from build123d import *

# Parameters (mm, degrees)
CYLINDER001_R     = 1.5
CYLINDER001_DEPTH = 10
CYLINDER_R        = 1.5
CYLINDER_DEPTH    = 10
EXTRUDE_DEPTH     = 12
BOX_W             = 31
BOX_H             = 12.3
BOX_DEPTH         = 0.75


with BuildPart() as screw_hole2:
    # Cylinder001 → Cylinder001 (new body)
    with BuildSketch(Plane(origin=(12.27, 0, 0), x_dir=(1, 0, 0), z_dir=(0, 0, 1))):
        Circle(CYLINDER001_R)
    extrude(amount=CYLINDER001_DEPTH)


with BuildPart() as screw_hole1:
    # Cylinder → Cylinder (new body)
    with BuildSketch(Plane(origin=(-12.27, 0, 0), x_dir=(1, 0, 0), z_dir=(0, 0, 1))):
        Circle(CYLINDER_R)
    extrude(amount=CYLINDER_DEPTH)


with BuildPart() as extrude_body:
    # Sketch → Extrude (new body)
    with BuildSketch(Plane.XY):
        with BuildLine():
            Line((-6.770935, 4.5), (6.770935, 4.5))
            ThreePointArc((9.25, 1.677142), (8.649385, 3.649675), (6.770935, 4.5))
            Line((9.25, 1.677142), (8.729065, -2.322858))
            ThreePointArc((6.25, -4.5), (7.899675, -3.878449), (8.729065, -2.322858))
            Line((6.25, -4.5), (-6.25, -4.5))
            ThreePointArc((-8.729065, -2.322858), (-7.899675, -3.878449), (-6.25, -4.5))
            Line((-8.729065, -2.322858), (-9.25, 1.677142))
            ThreePointArc((-6.770935, 4.5), (-8.649385, 3.649675), (-9.25, 1.677142))
        make_face()
    extrude(amount=EXTRUDE_DEPTH)


with BuildPart() as db9_connector:
    # Box → Box (new body)
    with BuildSketch(Plane(origin=(-15.5, -6.13, 6), x_dir=(1, 0, 0), z_dir=(0, 0, 1))):
        with Locations((15.5, 6.15)):
            Rectangle(BOX_W, BOX_H)
    extrude(amount=BOX_DEPTH)

    # Fusion: union Extrude body
    add(extrude_body.part)

    # Cut: cut screw_hole1
    add(screw_hole1.part, mode=Mode.SUBTRACT)

    # Cut001: cut screw_hole2
    add(screw_hole2.part, mode=Mode.SUBTRACT)


solid = db9_connector.part
Here's how the part is built. I have some questions about the finished solid (model axes, mm). A direction names the side the tool comes from. Round coordinates to 2 decimals unless told otherwise and drop trailing zeros. Loops run counter-clockwise (first coordinate to the right, second up) from the corner with the lowest first, then second, coordinate; pieces in that order, holes last. Notation, with made-up numbers: (-1, -33.5) -> (23, -33.5) arc R26 cw to (23, -14.5) -> close; hole circle Ø2 at (-37, 48). An arc over 180 degrees is marked (long way). Write each question's results on one line, items separated by ' | '.
(1) If I drill on L1, parallel to X at y = 0, z = 6.35; L2, parallel to Y at x = -12.27, z = 6.4; L3, parallel to Z at x = -10.5, y = 2.75, over which ranges is the centre line in solid material (lowest first)?
Worked answers:
L1: -15.5 to -13.77, -10.77 to 10.77, 13.77 to 15.5 | L2: -6.13 to -1.5, 1.5 to 6.17 | L3: 6 to 6.75
(2) If we section it at D-D, the plane y = 0.5: List the corners of the cut face in (x, z) for me, then the cut area to 3 significant figures.
Worked answers:
outline: (-15.5, 6) -> (-13.68, 6) -> (-13.68, 6.75) -> (-15.5, 6.75) -> close; (-10.86, 6) -> (-9.1, 6) -> (-9.1, 0) -> (9.1, 0) -> (9.1, 6) -> (10.86, 6) -> (10.86, 6.75) -> (9.1, 6.75) -> (9.1, 12) -> (-9.1, 12) -> (-9.1, 6.75) -> (-10.86, 6.75) -> close; (13.68, 6) -> (15.5, 6) -> (15.5, 6.75) -> (13.68, 6.75) -> close | area: 224 mm2
(3) We'd pull the mould along X, two halves only. Please class faces 1 (the face through (-10.884, -0.575, 6.37)), 2 (the face through (7.881, -3.895, 9.338)), 3 (the face through (-8.986, -0.351, 2.958)): released by +X, released by -X, zero draft, split by the parting line, or undercut.
Worked answers:
face 1: undercut | face 2: released by +X | face 3: released by -X
(4) If we section it at B-B, the plane x = 12.27: List the corners of the cut face in (y, z) for me, then the cut area to 4 significant figures.
Worked answers:
outline: (-6.13, 6) -> (-1.5, 6) -> (-1.5, 6.75) -> (-6.13, 6.75) -> close; (1.5, 6) -> (6.17, 6) -> (6.17, 6.75) -> (1.5, 6.75) -> close | area: 6.975 mm2
(5) For faces 4 (the face through (8.993, -0.295, 2.958)), 5 (the face through (-7.92, -3.86, 2.96)), 6 (the face through (-7.92, -3.86, 9.34)), which set-ups out of +Z, -Z, +X, -X, +Y, -Y let a thin tool reach every point of the face, with its end or its side?
Worked answers:
face 4: -Z, +X, -Y | face 5: -Z, -X, -Y | face 6: +Z, -X, -Y
(6) If we section it at C-C, the plane z = 7.25: List the corners of the cut face in (x, y) for me, then the cut area to 3 significant figures.
Worked answers:
outline: (-9.25, 1.68) -> (-8.73, -2.32) arc R2.5 ccw to (-6.25, -4.5) -> (6.25, -4.5) arc R2.5 ccw to (8.73, -2.32) -> (9.25, 1.68) arc R2.5 ccw to (6.77, 4.5) -> (-6.77, 4.5) arc R2.5 ccw to start | area: 157 mm2
(7) For P1, Ø4, axis at y = 3.5, z = 2, coming from the +X side; P2, Ø2.5, axis at x = -2, z = 9.5, coming from the +Y side; P3, Ø1.8, axis at x = -1.5, z = 2, coming from the -Y side, each with a flat end and sliding along its axis, tell me the tip position at first contact or that it passes through.
Worked answers:
P1: x = 9.27 | P2: y = 4.5 | P3: y = -4.5
(8) If we section it at A-A, the plane y = -3.5: List the corners of the cut face in (x, z) for me.
Worked answers:
outline: (-15.5, 6) -> (-8.25, 6) -> (-8.25, 0) -> (8.25, 0) -> (8.25, 6) -> (15.5, 6) -> (15.5, 6.75) -> (8.25, 6.75) -> (8.25, 12) -> (-8.25, 12) -> (-8.25, 6.75) -> (-15.5, 6.75) -> close
